from build123d import *

# Parameters (mm, degrees)
F1_DEPTH  = 210
F2_W      = 210
F2_H      = 20
F3_DEPTH  = 60
F4_DEPTH  = 60
F5_R      = 7
F6_DEPTH  = 50
F8_D      = 15
F8_DEPTH  = 40
F8_TIP    = 4.5064546427
F10_DEPTH = 20
F12_DEPTH = 20
F14_D     = 15
F14_DEPTH = 220
F14_TIP   = 4.5064546427
F15_W     = 20
F15_H     = 15
F16_DEPTH = 200
F17_D     = 10
F17_DEPTH = 40
F17_TIP   = 3.0043030951
F18_R     = 7
F19_DEPTH = 50


# Not quite as in the source:
# - a feature names something its author has since deleted; it is built from what else it names


with BuildPart() as f1:
    # F0 (on Front) → F1 (new body)
    with BuildSketch(Plane.XZ):
        with BuildLine():
            Line((0, 190), (0, 210))
            ThreePointArc((0, 210), (-148.4924240492, 148.4924240492), (-210, 0))
            Line((-210, 0), (-190, 0))
            ThreePointArc((-190, 0), (-134.3502884254, 134.3502884254), (0, 190))
        make_face()
    extrude(amount=F1_DEPTH)

    # F2 (on face) → F3 (join)
    with BuildSketch(Plane.YZ):
        with Locations((-105, 200)):
            Rectangle(F2_W, F2_H)
    extrude(amount=-F3_DEPTH)

    # F4 (add): a face of the model
    f4_faces = [f1.faces().sort_by_distance(p)[0] for p in [
        (-200, -105, 0),
    ]]
    extrude(f4_faces, amount=-F4_DEPTH)

    # F5 (on face) → F6 (cut)
    with BuildSketch(Plane.YZ):
        with Locations((-175, 200)):
            Circle(F5_R)
        with Locations((-140, 200)):
            Circle(F5_R)
        with Locations((-105, 200)):
            Circle(F5_R)
        with Locations((-70, 200)):
            Circle(F5_R)
        with Locations((-35, 200)):
            Circle(F5_R)
    extrude(amount=-F6_DEPTH, mode=Mode.SUBTRACT)

    # F8
    with Locations(Plane.XY.offset(210)):
        with Locations((-30, -157.5), (-30, -52.5)):
            Hole(F8_D / 2, depth=F8_DEPTH)
            with Locations((0, 0, -(F8_DEPTH + F8_TIP / 2))):  # 118° drill point
                Cone(0, F8_D / 2, F8_TIP, mode=Mode.SUBTRACT)

    # F9 (on face) → F10 (join)
    with BuildSketch(Plane.XZ.offset(210)):
        with BuildLine():
            ThreePointArc((-170, 0), (-120.2081528017, 120.2081528017), (0, 170))
            Line((0, 170), (0, 190))
            ThreePointArc((0, 190), (-134.3502884254, 134.3502884254), (-190, 0))
            Line((-190, 0), (-170, 0))
        make_face()
    extrude(amount=-F10_DEPTH)

    # F11 (on face) → F12 (join)
    with BuildSketch(Plane(origin=(0, 0, 0), x_dir=(-1, 0, 0), z_dir=(0, 1, 0))):
        with BuildLine():
            ThreePointArc((0, 170), (120.2081528017, 120.2081528017), (170, 0))
            Line((170, 0), (190, 0))
            ThreePointArc((190, 0), (134.3502884254, 134.3502884254), (0, 190))
            Line((0, 190), (0, 170))
        make_face()
    extrude(amount=-F12_DEPTH)

    # F14
    with Locations(Plane.XZ.offset(210)):
        with Locations((-183.5259069949, 49.1756185695), (-164.544826719, 95), (-134.3502884254, 134.3502884254), (-95, 164.544826719), (-49.1756185695, 183.5259069949)):
            Hole(F14_D / 2, depth=F14_DEPTH)
            with Locations((0, 0, -(F14_DEPTH + F14_TIP / 2))):  # 118° drill point
                Cone(0, F14_D / 2, F14_TIP, mode=Mode.SUBTRACT)

    # F15 (on face) → F16 (join)
    with BuildSketch(Plane(origin=(0, 0, 0), x_dir=(-1, 0, 0), z_dir=(0, 1, 0))):
        with Locations((30, 202.5)):
            Rectangle(F15_W, F15_H)
    extrude(amount=-F16_DEPTH)

    # F17
    with Locations(Plane.XY.offset(210)):
        with Locations((-30, -52.5), (-30, -157.5)):
            Hole(F17_D / 2, depth=F17_DEPTH)
            with Locations((0, 0, -(F17_DEPTH + F17_TIP / 2))):  # 118° drill point
                Cone(0, F17_D / 2, F17_TIP, mode=Mode.SUBTRACT)

    # F18 (on face) → F19 (cut)
    with BuildSketch(Plane(origin=(0, 0, 0), x_dir=(1, 0, 0), z_dir=(0, 0, -1))):
        with Locations((-200, 35)):
            Circle(F18_R)
        with Locations((-200, 70)):
            Circle(F18_R)
        with Locations((-200, 105)):
            Circle(F18_R)
        with Locations((-200, 140)):
            Circle(F18_R)
        with Locations((-200, 175)):
            Circle(F18_R)
    extrude(amount=-F19_DEPTH, mode=Mode.SUBTRACT)


solid = f1.part
CAD build for the part. Positions are in the model's coordinates, mm. A direction names the side the tool comes from. Round coordinates to 2 decimals unless told otherwise and drop trailing zeros. Write each loop counter-clockwise with the first axis right and the second up, starting at its lowest first coordinate (ties: lowest second). Pieces come first, ordered by that corner, then holes.
(1) Slice it at C-C, the plane x = -95. Write the cut outline in (y, z), and give its area (3 significant figures).
(2) 3-axis set-ups, long thin cutter, end or side, ignore diameter. For faces 5 (the face through (-31.6, -162.4, 195)), 6 (the face through (-60, -106, 206)), 7 (the face through (-50, -140, 200)): which of +Z, -Z, +X, -X, +Y, -Y reach the whole face in a straight line?
(3) Slice it at A-A, the plane z = 46. Write the cut outline in (x, y).
(4) Drop flat-ended pins along their axis: P1, Ø18, axis at y = -105, z = 200, coming from the +X side; P2, Ø6, axis at y = -176, z = 202, coming from the +X side; P3, Ø1.5, axis at x = -99.5, y = -47.5, coming from the +Z side; P4, Ø12, axis at y = -128.5, z = 115.5, coming from the -X side. Give the stop position or say it passes through.
(5) Probe line 1 along Y through (x, z) = (-200, 10); line 2 along Y through (x, z) = (-30, 200); line 3 along X through (y, z) = (-140, 49). List the from-to ranges inside material, lowest first.
(6) Mould opens along Y. For faces 1 (the face through (-120, 0, 129)), 2 (the face through (-37.154, -155.247, 191.541)), 3 (the face through (-147.46, -103.53, 149.52)), 4 (the face through (-193.534, -172.319, 24.65)) say: pulls with the +Y half, pulls with the -Y half, needs draft (parallel to the pull), parting line crosses it, or undercut.
(7) Slice it at D-D, the plane z = 95. Write the cut outline in (x, y), and give its area (3 significant figures).
From the geometry:
1. outline: (-210, 140.98) - (-190, 140.98) - (-190, 157.04) - (-210, 157.04) - close; (-210, 172.04) - (0, 172.04) - (0, 187.28) - (-210, 187.28) - close; (-20, 140.98) - (0, 140.98) - (0, 157.04) - (-20, 157.04) - close
1. area: 3,840 mm2
2. face 5: -Z
2. face 6: +Z, -X, +Y, -Y
2. face 7: none
3. outline: (-210, -210) - (-190.32, -210) - (-190.32, 0) - (-210, 0) - close; (-176.73, -210) - (-163.66, -210) - (-163.66, -190) - (-176.73, -190) - close; (-176.73, -20) - (-163.66, -20) - (-163.66, 0) - (-176.73, 0) - close; hole circle Ø14 at (-200, -175); hole circle Ø14 at (-200, -140); hole circle Ø14 at (-200, -105); hole circle Ø14 at (-200, -70); hole circle Ø14 at (-200, -35)
4. P1: stops at x = 0
4. P2: stops at x = -20
4. P3: stops at z = 185.33
4. P4: stops at x = -179.19
5. line 1: y = -210 to -182, -168 to -147, -133 to -112, -98 to -77, -63 to -42, -28 to 0
5. line 2: y = -210 to -162.5, -152.5 to -57.5, -47.5 to 0
5. line 3: x = -210 to -207, -193 to -191.02
6. face 1: pulls with the +Y half
6. face 2: undercut
6. face 3: needs draft
6. face 4: undercut
7. outline: (-187.28, -210) - (-172.04, -210) - (-172.04, 0) - (-187.28, 0) - close; (-157.04, -210) - (-140.98, -210) - (-140.98, -190) - (-157.04, -190) - close; (-157.04, -20) - (-140.98, -20) - (-140.98, 0) - (-157.04, 0) - close
7. area: 3,840 mm2
